```python
from build123d import *

# Parameters (mm, degrees)
SKETCH1_R           = 57.5
SKETCH1_R_2         = 40
SKETCH1_R_3         = 1.5
BOSS_EXTRUDE1_DEPTH = 14
SKETCH2_R           = 42.5
SKETCH2_R_2         = 36
BOSS_EXTRUDE2_DEPTH = 9
SKETCH3_R           = 1.5
CUT_EXTRUDE1_DEPTH  = 5


with BuildPart() as part:
    # Sketch1 → Boss-Extrude1 (new body)
    with BuildSketch(Plane(origin=(0, 0, 0), x_dir=(1, 0, 0), z_dir=(0, 1, 0))):
        with Locations(Location((0, 0, 0), (0, 0, 270))):
            Circle(SKETCH1_R)
        with Locations(Location((0, 0, 0), (0, 0, 270))):
            Circle(SKETCH1_R_2, mode=Mode.SUBTRACT)
        with Locations(Location((0, 55, 0), (0, 0, 270))):
            Circle(SKETCH1_R_3, mode=Mode.SUBTRACT)
        with Locations(Location((27.5, 47.631397208, 0), (0, 0, 270))):
            Circle(SKETCH1_R_3, mode=Mode.SUBTRACT)
        with Locations(Location((47.631397208, 27.5, 0), (0, 0, 270))):
            Circle(SKETCH1_R_3, mode=Mode.SUBTRACT)
        with Locations(Location((55, 0, 0), (0, 0, 270))):
            Circle(SKETCH1_R_3, mode=Mode.SUBTRACT)
        with Locations(Location((47.631397208, -27.5, 0), (0, 0, 270))):
            Circle(SKETCH1_R_3, mode=Mode.SUBTRACT)
        with Locations(Location((27.5, -47.631397208, 0), (0, 0, 270))):
            Circle(SKETCH1_R_3, mode=Mode.SUBTRACT)
        with Locations(Location((0, -55, 0), (0, 0, 270))):
            Circle(SKETCH1_R_3, mode=Mode.SUBTRACT)
        with Locations(Location((-27.5, -47.631397208, 0), (0, 0, 270))):
            Circle(SKETCH1_R_3, mode=Mode.SUBTRACT)
        with Locations(Location((-47.631397208, -27.5, 0), (0, 0, 270))):
            Circle(SKETCH1_R_3, mode=Mode.SUBTRACT)
        with Locations(Location((-55, 0, 0), (0, 0, 270))):
            Circle(SKETCH1_R_3, mode=Mode.SUBTRACT)
        with Locations(Location((-47.631397208, 27.5, 0), (0, 0, 270))):
            Circle(SKETCH1_R_3, mode=Mode.SUBTRACT)
        with Locations(Location((-27.5, 47.631397208, 0), (0, 0, 270))):
            Circle(SKETCH1_R_3, mode=Mode.SUBTRACT)
    extrude(amount=BOSS_EXTRUDE1_DEPTH)

    # Sketch2 → Boss-Extrude2 (add)
    with BuildSketch(Plane(origin=(0, 14, 0), x_dir=(1, 0, 0), z_dir=(0, 1, 0))):
        Circle(SKETCH2_R)
        with Locations(Location((0, 0, 0), (0, 0, 270))):
            Circle(SKETCH2_R_2, mode=Mode.SUBTRACT)
    extrude(amount=-BOSS_EXTRUDE2_DEPTH)

    # Sketch3 → Cut-Extrude1 (cut)
    with BuildSketch(Plane.XZ):
        with Locations(Location((0, 45, 0), (0, 0, 270))):
            Circle(SKETCH3_R)
        with Locations(Location((24.328836786, 37.856408977, 0), (0, 0, 270))):
            Circle(SKETCH3_R)
        with Locations(Location((40.933439791, 18.693675585, 0), (0, 0, 270))):
            Circle(SKETCH3_R)
        with Locations(Location((44.541964885, -6.404167722, 0), (0, 0, 270))):
            Circle(SKETCH3_R)
        with Locations(Location((34.008730846, -29.468733028, 0), (0, 0, 270))):
            Circle(SKETCH3_R)
        with Locations(Location((12.677965058, -43.177183813, 0), (0, 0, 270))):
            Circle(SKETCH3_R)
        with Locations(Location((-12.677965058, -43.177183813, 0), (0, 0, 270))):
            Circle(SKETCH3_R)
        with Locations(Location((-34.008730846, -29.468733028, 0), (0, 0, 270))):
            Circle(SKETCH3_R)
        with Locations(Location((-44.541964885, -6.404167722, 0), (0, 0, 270))):
            Circle(SKETCH3_R)
        with Locations(Location((-40.933439791, 18.693675585, 0), (0, 0, 270))):
            Circle(SKETCH3_R)
        with Locations(Location((-24.328836786, 37.856408977, 0), (0, 0, 270))):
            Circle(SKETCH3_R)
    extrude(amount=-CUT_EXTRUDE1_DEPTH, mode=Mode.SUBTRACT)


solid = part.part
```
Can you work these out from the model? Positions are in its coordinate system, mm. A direction names the side the tool comes from. Give positions to 0.01 mm unless a question says otherwise; leave off trailing zeros. Loops run counter-clockwise (first coordinate to the right, second up) from the corner with the lowest first, then second, coordinate; pieces in that order, holes last. Notation, with made-up numbers: M -6.75,-16 L 14.25,-16 A7 ccw 14.25,-6 Z; hole C -7.5,31.25 d1. An arc over 180 degrees is marked long. Use one line per item in the form item = value. Start each with the question number.
(1) I want a section at C-C, the plane y = 11.5. State how many separate pieces and enclosed holes the cut face has, and give its area (3 significant figures).
(2) I want a section at B-B, the plane x = 27.5. Write out the boundary of the cut face in (y, z), and give its area (3 significant figures).
(3) I'm going to push flat-ended pins straight in: P1, Ø6, axis at x = 21, y = 11, coming from the -Z side; P2, Ø1.5, axis at x = 33.5, z = -29, coming from the -Y side; P3, Ø3, axis at x = 18, y = 11, coming from the +Z side. Where does each tip first touch, or does it pass through?
(4) I want a section at D-D, the plane z = -55. Write out the boundary of the cut face in (x, y), and give its area (3 significant figures).
(5) Thinking about a two-plate mould opening in X: for faces 3 (the cylindrical face through (10.81, 9.56, 34.34)), 4 (the cylindrical face through (-56.133, 6.902, -12.465)), which applies, released by +X, released by -X, zero draft, split by the parting line, or undercut?
(6) On a 3-axis mill with a long thin cutter (end or side, diameter ignored), from which of +Z, -Z, +X, -X, +Y, -Y can I reach the whole of each face in a straight line? I mean faces 1 (the cylindrical face through (-43.528, 2.465, -5.299)), 2 (the cylindrical face through (28.987, 6.902, -47.827)). Say none if no direction works.
(7) Please list where these lines run through material, in increasing order: line 1 (X direction, y = 2.25, z = 0); line 2 (X direction, y = 9.75, z = -0.5); line 3 (Z direction, x = -12.5, y = 4.75).
(8) I want a section at A-A, the plane z = 27.5. Write out the boundary of the cut face in (x, y).
Worked out:
q1.separate_pieces = 1
q1.enclosed_holes = 13
q1.area = 6,230 mm²
q2.outline = M 0,-50.5 L 14,-50.5 L 14,-49.13 L 0,-49.13 Z; M 0,-46.13 L 14,-46.13 L 14,-23.23 L 5,-23.23 L 5,-29.05 L 0,-29.05 Z; M 0,29.05 L 5,29.05 L 5,23.23 L 14,23.23 L 14,46.13 L 0,46.13 Z; M 0,49.13 L 14,49.13 L 14,50.5 L 0,50.5 Z
q2.area = 621 mm²
q3.P1 = -54.61
q3.P2 = 5
q3.P3 = 55.08
q4.outline = M -16.77,0 L -1.5,0 L -1.5,14 L -16.77,14 Z; M 1.5,0 L 16.77,0 L 16.77,14 L 1.5,14 Z
q4.area = 428 mm²
q5.face_3 = undercut
q5.face_4 = split by the parting line
q6.face_1 = -Y
q6.face_2 = +Y, -Y
q7.line_1 = -57.5 to -56.5, -53.5 to -40, 40 to 53.5, 56.5 to 57.5
q7.line_2 = -57.5 to -56.41, -53.59 to -36, 36 to 53.59, 56.41 to 57.5
q7.line_3 = -56.12 to -44.67, -41.69 to -38, 38 to 56.12
q8.outline = M -50.5,0 L -49.13,0 L -49.13,14 L -50.5,14 Z; M -46.13,0 L -29.05,0 L -29.05,5 L -23.23,5 L -23.23,14 L -46.13,14 Z; M 23.23,5 L 29.05,5 L 29.05,0 L 46.13,0 L 46.13,14 L 23.23,14 Z; M 49.13,0 L 50.5,0 L 50.5,14 L 49.13,14 Z
